from build123d import *

# Parameters (mm, degrees)
SKETCH1_W           = 50
SKETCH1_H           = 420
BOSS_EXTRUDE1_DEPTH = 150
CUT_EXTRUDE1_DEPTH  = 447.68221366
SKETCH4_W           = 5
SKETCH4_H           = 150
BOSS_EXTRUDE2_DEPTH = 50
SKETCH5_W           = 5
SKETCH5_H           = 150
BOSS_EXTRUDE3_DEPTH = 50
SKETCH7_W           = 5
SKETCH7_H           = 150
BOSS_EXTRUDE4_DEPTH = 50
SKETCH8_W           = 5
SKETCH8_H           = 150
BOSS_EXTRUDE5_DEPTH = 50


with BuildPart() as part:
    # Sketch1 → Boss-Extrude1 (new body)
    with BuildSketch(Plane(origin=(0, 0, 0), x_dir=(1, 0, 0), z_dir=(0, 1, 0))):
        with Locations((0, 210)):
            Rectangle(SKETCH1_W, SKETCH1_H)
    extrude(amount=BOSS_EXTRUDE1_DEPTH)

    # Sketch3 → Cut-Extrude1 (cut, through all)
    with BuildSketch(Plane.XY):
        Polygon((-20, 75), (-20, 5), (20, 5), (20, 145), (-20, 145), align=None)
    extrude(amount=-CUT_EXTRUDE1_DEPTH, mode=Mode.SUBTRACT)

    # Sketch4 → Boss-Extrude2 (add)
    with BuildSketch(Plane.XY):
        with Locations((22.5, 75)):
            Rectangle(SKETCH4_W, SKETCH4_H)
    extrude(amount=BOSS_EXTRUDE2_DEPTH)

    # Sketch5 → Boss-Extrude3 (add)
    with BuildSketch(Plane.XY):
        with Locations((-22.5, 75)):
            Rectangle(SKETCH5_W, SKETCH5_H)
    extrude(amount=BOSS_EXTRUDE3_DEPTH)

    # Sketch7 → Boss-Extrude4 (add)
    with BuildSketch(Plane(origin=(0, 0, -420), x_dir=(-1, 0, 0), z_dir=(0, 0, -1))):
        with Locations((-22.5, 75)):
            Rectangle(SKETCH7_W, SKETCH7_H)
    extrude(amount=BOSS_EXTRUDE4_DEPTH)

    # Sketch8 → Boss-Extrude5 (add)
    with BuildSketch(Plane(origin=(0, 0, -420), x_dir=(-1, 0, 0), z_dir=(0, 0, -1))):
        with Locations((22.5, 75)):
            Rectangle(SKETCH8_W, SKETCH8_H)
    extrude(amount=BOSS_EXTRUDE5_DEPTH)


solid = part.part
Read the model definition and answer for the solid it produces. Units are mm, in the model's axes. A direction names the side the tool comes from. Give positions to 0.01 mm unless a question says otherwise; leave off trailing zeros. Write each loop counter-clockwise with the first axis right and the second up, starting at its lowest first coordinate (ties: lowest second). Pieces come first, ordered by that corner, then holes. Notation, with made-up numbers: (16.25, 52.5) - (36.25, 52.5) arc R24 ccw to (36.25, 65.5) - close; hole circle Ø6 at (29, 40.5). An arc over 180 degrees is marked (long way). Return JSON: item names as keys, results as strings.
Q1. A cutting plane is placed at A-A, the plane y = 20.5. Determine the outline of the cut face in (x, z), and give its area (3 significant figures).
Reply:
{"outline": "(-25, -470) - (-20, -470) - (-20, 50) - (-25, 50) - close; (20, -470) - (25, -470) - (25, 50) - (20, 50) - close", "area": "5,200 mm²"}
Q2. For a pull along Y with two mould halves and no side action, classify faces 1 (the face through (20, 74, -206)), 2 (the face through (25, 74, -206)), 3 (the face through (0, 0, -206)) as released by +Y, released by -Y, zero draft, split by the parting line, or undercut.
Reply:
{"face 1": "undercut", "face 2": "zero draft", "face 3": "released by -Y"}
Q3. A cutting plane is placed at B-B, the plane x = 4. Determine the outline of the cut face in (y, z), and give its area (3 significant figures).
Reply:
{"outline": "(0, -420) - (5, -420) - (5, 0) - (0, 0) - close; (145, -420) - (150, -420) - (150, 0) - (145, 0) - close", "area": "4,200 mm²"}
Q4. Given P1, Ø4, axis at x = -16.5, z = -298, coming from the -Y side; P2, Ø1.5, axis at x = -3.5, y = 2.5, coming from the +Z side; P3, Ø5.5, axis at x = 0.5, y = 3.5, coming from the -Z side, each flat-ended and moving along its own axis, determine where each tip first touches the part or whether it passes through.
Reply:
{"P1": "y = 0", "P2": "z = 0", "P3": "z = -420"}
Q5. A cutting plane is placed at C-C, the plane z = -402.5. Determine the outline of the cut face in (x, y).
Reply:
{"outline": "(-25, 0) - (25, 0) - (25, 150) - (-25, 150) - close; hole (-20, 5) - (20, 5) - (20, 145) - (-20, 145) - close"}
Q6. Consider line 1 along X through (y, z) = (96, -125.5); line 2 along Y through (x, z) = (3.5, -212.5). Determine where each line is inside the solid, lowest interval first. Write a range as [from, to].
Reply:
{"line 1": "[-25, -20], [20, 25]", "line 2": "[0, 5], [145, 150]"}
Q7. For faces 4 (the face through (0, 5, -207)), 5 (the face through (-25, 74, -206)), determine the directions among +Z, -Z, +X, -X, +Y, -Y from which every point of the face is accessible in a straight line to the end or side of a thin tool.
Reply:
{"face 4": "+Z, -Z", "face 5": "+Z, -Z, -X, +Y, -Y"}
